```python
from build123d import *

# Parameters (mm, degrees)
BOSS_EXTRUDE1_DEPTH = 19
SKETCH1_3_R         = 1.1
CUT_EXTRUDE1_DEPTH  = 5
CUT_EXTRUDE1_TAPER  = 6


with BuildPart() as part:
    # Sketch1 → Boss-Extrude1 (new body)
    with BuildSketch(Plane.YZ):
        with BuildLine():
            Line((1, 0), (3.2, 0))
            ThreePointArc((3.2, 0), (3.907106781, 0.292893219), (4.2, 1))
            Line((4.2, 1), (4.2, 3.2))
            ThreePointArc((4.2, 3.2), (3.907106781, 3.907106781), (3.2, 4.2))
            Line((3.2, 4.2), (1, 4.2))
            ThreePointArc((1, 4.2), (0.292893219, 3.907106781), (0, 3.2))
            Line((0, 3.2), (0, 1))
            ThreePointArc((0, 1), (0.292893219, 0.292893219), (1, 0))
        make_face()
    extrude(amount=BOSS_EXTRUDE1_DEPTH)

    # Sketch1<3> → Cut-Extrude1 (cut)
    with BuildSketch(Plane.YZ):
        with Locations((2.1, 2.1)):
            Circle(SKETCH1_3_R)
    cut_extrude1 = extrude(amount=CUT_EXTRUDE1_DEPTH, taper=CUT_EXTRUDE1_TAPER, mode=Mode.SUBTRACT)

    # Mirror1: Cut-Extrude1 across plane
    add(cut_extrude1.mirror(Plane(origin=(9.5, 0, 0), x_dir=(0, 0, 1), z_dir=(1, 0, 0))), mode=Mode.SUBTRACT)


solid = part.part
```
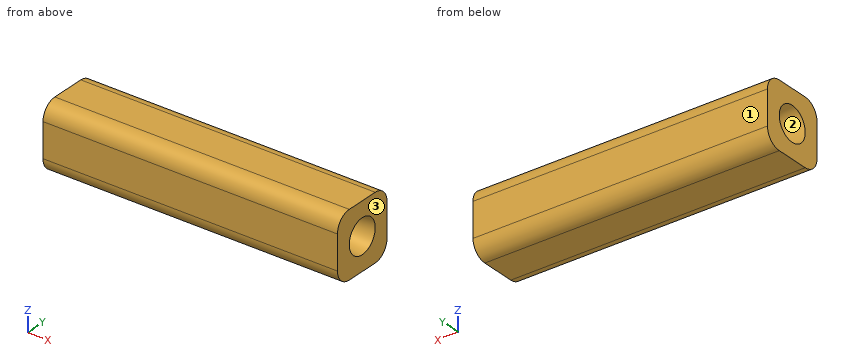
Geometry: final body of the model. Coordinates: model frame, mm. Face numbers are marked on the shaded views. Give positions to 0.01 mm unless a question says otherwise; leave off trailing zeros. Loops run counter-clockwise (first coordinate to the right, second up) from the corner with the lowest first, then second, coordinate; pieces in that order, holes last. Notation, with made-up numbers: (64, 18) -> (123, 18) arc R23 cw to (123, 28) -> close; hole circle Ø7 at (70, -7). An arc over 180 degrees is marked (long way). Use one line per item in the form item = value.
Item 1: Section query A-A on x = 11. Output: boundary loops of the cut face in (y, z), and give its area (3 significant figures).
A:
outline = (0, 1) arc R1 ccw to (1, 0) -> (3.2, 0) arc R1 ccw to (4.2, 1) -> (4.2, 3.2) arc R1 ccw to (3.2, 4.2) -> (1, 4.2) arc R1 ccw to (0, 3.2) -> close
area = 16.8 mm^2
Item 2: Section query D-D on z = 3.5. Output: boundary loops of the cut face in (x, y), and give its area (3 significant figures).
A:
outline = (0, 0.05) -> (19, 0.05) -> (19, 4.15) -> (0, 4.15) -> close
area = 78.0 mm^2
Item 3: Line query: probe 1 along Z at (x, y) = (1, 2.05); probe 2 along Y at (x, z) = (4.75, 2.45); probe 3 along Y at (x, z) = (17.75, 0.85). Output: solid intervals per line, ascending.
A:
probe_1 = 0 to 1.11, 3.09 to 4.2
probe_2 = 0 to 1.61, 2.59 to 4.2
probe_3 = 0.01 to 4.19
Item 4: Draft query along Y for the marked faces 1, 2 and 3. Return one class per face: pulls with the +Y half, pulls with the -Y half, needs draft (parallel to the pull), parting line crosses it, or undercut.
A:
face_1 = pulls with the +Y half
face_2 = undercut
face_3 = needs draft
Item 5: Section query B-B on y = 2.1. Output: boundary loops of the cut face in (x, z).
A:
outline = (0, 0) -> (19, 0) -> (19, 1) -> (14, 1.53) -> (14, 2.67) -> (19, 3.2) -> (19, 4.2) -> (0, 4.2) -> (0, 3.2) -> (5, 2.67) -> (5, 1.53) -> (0, 1) -> close
Item 6: Section query C-C on x = 3.5. Output: boundary loops of the cut face in (y, z).
A:
outline = (0, 1) arc R1 ccw to (1, 0) -> (3.2, 0) arc R1 ccw to (4.2, 1) -> (4.2, 3.2) arc R1 ccw to (3.2, 4.2) -> (1, 4.2) arc R1 ccw to (0, 3.2) -> close; hole circle Ø1.46 at (2.1, 2.1)
